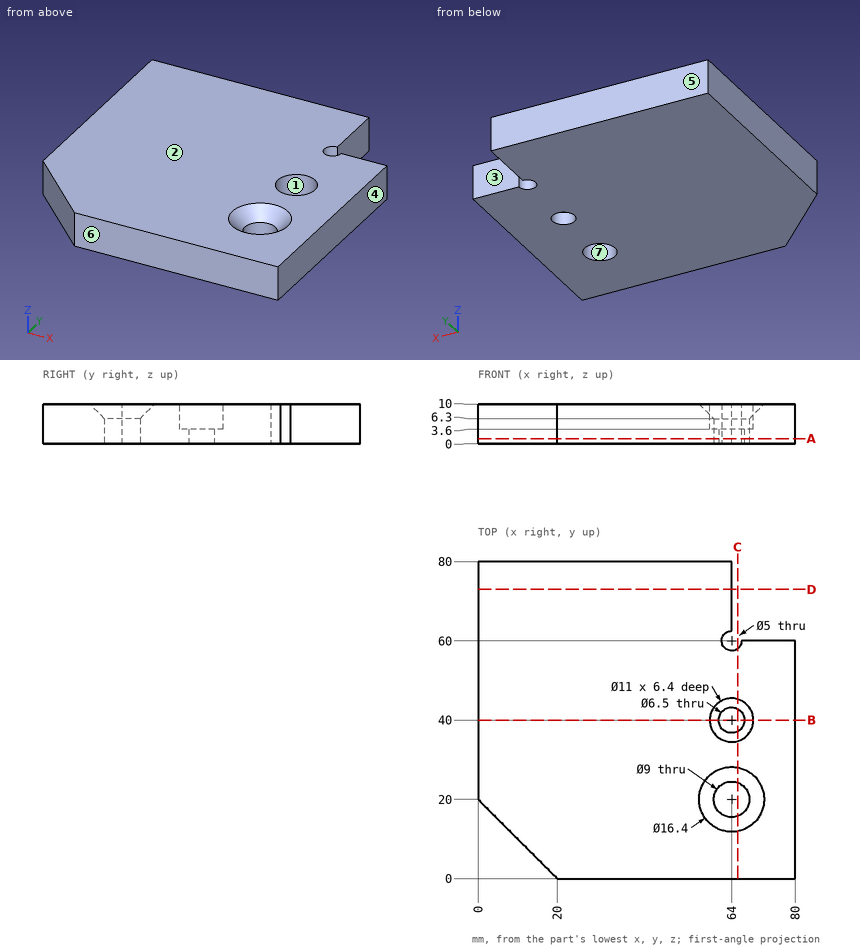
Geometry: see drawing. Coordinates: mm, zero at the bounding-box minimum. A direction names the side the tool comes from. Coordinates: 2 decimals unless noted, no trailing zeros. Order: outer loops, then holes, each group sorted by start corner. A loop starts at its lowest first (then second) coordinate and runs counter-clockwise, first axis right, second up. Notation, with made-up numbers: M -31,-37 L -13,-37 A13 cw -13,-18 Z; hole C -11,89 d7. An arc over 180 degrees is marked long. Write item = value, one per line. Start each with the question number.
(1) Section C-C on x = 65.5. Give the number of separate pieces and of enclosed holes in the cut face, and give its area (3 significant figures).
(2) Pull-direction query (Y, two-part tool) for the marked faces 4, 5, 6 and 7; classes: released by +Y, released by -Y, zero draft, split by the parting line, or undercut.
(3) Line query: line 1 along Y through (x, z) = (73, 1); line 2 along X through (y, z) = (39.5, 7); line 3 along X through (y, z) = (63, 2.25). Output: solid intervals per line, ascending. Write a range as [from, to].
(4) Section B-B on y = 40. Output: boundary loops of the cut face in (x, z), and give its area (3 significant figures).
(5) Section A-A on z = 1.25. Output: boundary loops of the cut face in (x, y), and give its area (3 significant figures).
(6) Reachability of the marked faces 1, 2 and 3 from +Z, -Z, +X, -X, +Y, -Y: full face, straight path, thin tool, end or side. Return the list, or none.
(7) Section D-D on y = 73. Output: boundary loops of the cut face in (x, z), and give its area (3 significant figures).
(8) First-contact query: P1, Ø6, axis at x = 64, y = 60, coming from the +Z side; P2, Ø5.5, axis at x = 64, y = 20, coming from the -Z side. Flat tips, straight axial feed; report the tip coordinate or a pass-through.
Result set:
q1.separate_pieces = 3
q1.enclosed_holes = 0
q1.area = 392 mm²
q2.face_4 = zero draft
q2.face_5 = released by +Y
q2.face_6 = released by -Y
q2.face_7 = undercut
q3.line_1 = [0, 60]
q3.line_2 = [0, 58.52], [69.48, 80]
q3.line_3 = [0, 64]
q4.outline = M 0,0 L 60.75,0 L 60.75,3.6 L 58.5,3.6 L 58.5,10 L 0,10 Z; M 67.25,0 L 80,0 L 80,10 L 69.5,10 L 69.5,3.6 L 67.25,3.6 Z
q4.area = 706 mm²
q5.outline = M 0,20 L 20,0 L 80,0 L 80,60 L 66.5,60 A2.5 cw long 64,62.5 L 64,80 L 0,80 Z; hole C 64,20 d9; hole C 64,40 d6.5
q5.area = 5,770 mm²
q6.face_1 = +Z
q6.face_2 = +Z, +X, -X, +Y, -Y
q6.face_3 = +Z, -Z, +X, +Y
q7.outline = M 0,0 L 64,0 L 64,10 L 0,10 Z
q7.area = 640 mm²
q8.P1 = 10
q8.P2 = through
